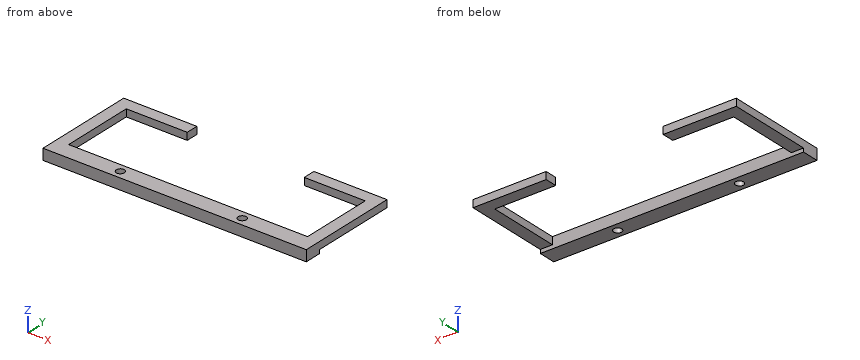
Autodesk Fusion 360 part; units mm, degrees
sketch "Sketch1" plane through (0, 0, 0) normal (0, 0, 1) x (1, 0, 0)
  line L0 (54, 3.5) -> (-54, 3.5)
  line L1 (-54, 3.5) -> (-54, -3.5)
  line L2 (-54, -3.5) -> (54, -3.5)
  line L3 (54, -3.5) -> (54, 3.5)
  line L4 (54, 3.5) -> (-54, -3.5) construction
  line L5 (-54, 3.5) -> (54, -3.5) construction
  circle A0 centre (-25, 0) radius 1.675
  line L6 (0, 3.5) -> (0, -3.5) construction
  circle A1 centre (25, 0) radius 1.675
  dimension "d1" = 108
  dimension "width" = 7
  dimension "d3" = 3.35
  dimension "d21" = 25
extrude "Extrude1" add sketch "Sketch1" along normal blind 4.5
sketch "Sketch2" plane through (0, 3.5, 0) normal (0, 1, 0) x (-1, 0, 0)
  line L0 (-54, 0) -> (54, 0)
  line L1 (54, 0) -> (54, 4.5)
  line L2 (54, 4.5) -> (-54, 4.5)
  line L3 (-54, 4.5) -> (-54, 0)
  line L4 (-54, 4.5) -> (-49, 4.5)
  line L5 (-49, 4.5) -> (-49, 1.5)
  line L6 (-49, 1.5) -> (-54, 1.5)
  line L7 (-54, 1.5) -> (-54, 4.5)
  line L8 (0, 4.5) -> (0, 0) construction
  line L9 (49, 4.5) -> (49, 1.5)
  line L10 (49, 1.5) -> (54, 1.5)
  line L11 (54, 1.5) -> (54, 4.5)
  line L12 (54, 4.5) -> (49, 4.5)
  dimension "d6" = 5
extrude "Extrude2" add sketch "Sketch2" along normal blind 35 contours L2 L3 L4 L5 L6 L7 | L1 L2 L9 L10 L11 L12
sketch "Sketch3" plane through (-49, 0, 0) normal (1, 0, 0) x (0, 1, 0)
  line L0 (3.5, 4.5) -> (3.5, 1.5)
  line L1 (3.5, 1.5) -> (38.5, 1.5)
  line L2 (38.5, 1.5) -> (38.5, 4.5)
  line L3 (38.5, 4.5) -> (3.5, 4.5)
  line L4 (38.5, 4.5) -> (33.5, 4.5)
  line L5 (33.5, 4.5) -> (33.5, 1.5)
  line L6 (33.5, 1.5) -> (38.5, 1.5)
  line L7 (38.5, 1.5) -> (38.5, 4.5)
  dimension "d9" = 5
sketch "Sketch4" plane through (49, 0, 0) normal (-1, 0, 0) x (0, -1, 0)
  line L0 (-3.5, 1.5) -> (-3.5, 4.5)
  line L1 (-3.5, 4.5) -> (-38.5, 4.5)
  line L2 (-38.5, 4.5) -> (-38.5, 1.5)
  line L3 (-38.5, 1.5) -> (-3.5, 1.5)
  line L4 (-38.5, 4.5) -> (-33.5, 4.5)
  line L5 (-33.5, 4.5) -> (-33.5, 1.5)
  line L6 (-33.5, 1.5) -> (-38.5, 1.5)
  line L7 (-38.5, 1.5) -> (-38.5, 4.5)
  dimension "d10" = 5
extrude "Extrude3" add sketch "Sketch4" along normal blind 25 contours L1 L2 L3 L4 L5 L6 L7
extrude "Extrude4" add sketch "Sketch3" along normal blind 25 contours L1 L2 L3 L4 L5 L6 L7
sketch "Sketch5" plane through (0, 0, 4.5) normal (0, 0, 1) x (-1, 0, 0)
  circle A0 centre (25, 0) radius 1.675
  circle A1 centre (-25, 0) radius 1.675
  line L0 (-54, 3.5) -> (-54, -38.5)
  line L1 (-54, -38.5) -> (-24, -38.5)
  line L2 (-24, -38.5) -> (-24, -33.5)
  line L3 (-24, -33.5) -> (-49, -33.5)
  line L4 (-49, -33.5) -> (-49, -3.5)
  line L5 (-49, -3.5) -> (49, -3.5)
  line L6 (49, -3.5) -> (49, -33.5)
  line L7 (49, -33.5) -> (24, -33.5)
  line L8 (24, -33.5) -> (24, -38.5)
  line L9 (24, -38.5) -> (54, -38.5)
  line L10 (54, -38.5) -> (54, 3.5)
  line L11 (54, 3.5) -> (-54, 3.5)
  line L12 (-24, -36) -> (-54, -36) construction
extrude "Extrude5" [suppressed]
Geometry check sheet. Reference: the model listing, model coordinates, mm. Give positions to 0.01 mm unless a question says otherwise; leave off trailing zeros. Loops run counter-clockwise (first coordinate to the right, second up) from the corner with the lowest first, then second, coordinate; pieces in that order, holes last.
(1) Thickness scan on L1, parallel to Y at x = -25, z = 2.85 (3 decimals); L2, parallel to X at y = 7, z = 3.9; L3, parallel to X at y = 1.5, z = 1.5. Record the ranges inside material, lowest first.
From the geometry:
L1: y = -3.5 to -1.675, 1.675 to 3.5, 33.5 to 38.5
L2: x = -54 to -49, 49 to 54
L3: x = -54 to -25.75, -24.25 to 24.25, 25.75 to 54
(2) Section check A-A on y = 0. Record the cut outline in (x, z) (3 decimals).
From the geometry:
outline: (-54, 0) - (-26.675, 0) - (-26.675, 4.5) - (-54, 4.5) - close; (-23.325, 0) - (23.325, 0) - (23.325, 4.5) - (-23.325, 4.5) - close; (26.675, 0) - (54, 0) - (54, 4.5) - (26.675, 4.5) - close
(3) Depth check by flat-ended pin: pin 1 Ø24 at (x, y) = (-33.5, 25.5) entering from -Z. Enter the tip coordinate at first touch or a pass-through.
From the geometry:
pin 1: stops at z = 1.5
(4) Section check C-C on y = 13. Record the cut outline in (x, z).
From the geometry:
outline: (-54, 1.5) - (-49, 1.5) - (-49, 4.5) - (-54, 4.5) - close; (49, 1.5) - (54, 1.5) - (54, 4.5) - (49, 4.5) - close
(5) Section check D-D on x = 36. Record the cut outline in (y, z).
From the geometry:
outline: (-3.5, 0) - (3.5, 0) - (3.5, 4.5) - (-3.5, 4.5) - close; (33.5, 1.5) - (38.5, 1.5) - (38.5, 4.5) - (33.5, 4.5) - close
(6) Section check B-B on x = -25. Record the cut outline in (y, z) (3 decimals), then the cut area to 3 significant figures.
From the geometry:
outline: (-3.5, 0) - (-1.675, 0) - (-1.675, 4.5) - (-3.5, 4.5) - close; (1.675, 0) - (3.5, 0) - (3.5, 4.5) - (1.675, 4.5) - close; (33.5, 1.5) - (38.5, 1.5) - (38.5, 4.5) - (33.5, 4.5) - close
area: 31.4 mm2
